from build123d import *

# Parameters (mm, degrees)
SKETCH1_R           = 28.575
SKETCH1_R_2         = 12.7
SKETCH1_R_3         = 3.175
BOSS_EXTRUDE1_DEPTH = 6.35


with BuildPart() as part:
    # Sketch1 → Boss-Extrude1 (new body)
    with BuildSketch(Plane.ZY.offset(-33.3375)):
        with Locations((-3.206573009, 186.931527045)):
            Circle(SKETCH1_R)
        with Locations((-3.206573009, 186.931527045)):
            Circle(SKETCH1_R_2, mode=Mode.SUBTRACT)
        with Locations((19.018426991, 186.931527045)):
            Circle(SKETCH1_R_3, mode=Mode.SUBTRACT)
        with Locations((-3.206573009, 164.706527045)):
            Circle(SKETCH1_R_3, mode=Mode.SUBTRACT)
        with Locations((-25.431573009, 186.931527045)):
            Circle(SKETCH1_R_3, mode=Mode.SUBTRACT)
        with Locations((-3.206573009, 209.156527045)):
            Circle(SKETCH1_R_3, mode=Mode.SUBTRACT)
    extrude(amount=BOSS_EXTRUDE1_DEPTH)


solid = part.part
For this review, take the finished solid that the model builds, in its own axes (mm). Round coordinates to 2 decimals unless told otherwise and drop trailing zeros. Write each loop counter-clockwise with the first axis right and the second up, starting at its lowest first coordinate (ties: lowest second). Pieces come first, ordered by that corner, then holes. Notation, with made-up numbers: M 41.25,12 L 76.25,12 A27 cw 76.25,50 Z; hole C -36.5,21.25 d3. An arc over 180 degrees is marked long. Write item = value, one per line. Start each with the question number.
(1) We need section D-D (x = 29.5). Give the boundary of the cut face in (y, z) (3 decimals), then the cut area to 3 significant figures.
(2) The part is to be moulded in two halves that separate along Z. For faces 1 (the face through (33.338, 175, 3)), 2 (the face through (30.207, 211.026, 12.155)), 3 (the face through (30.207, 187.885, 22.047)), say which applies: +Z half, -Z half, draft (parallel to the pull), parting line (faces both ways), or undercut.
(3) For line 1 along Y through (x, z) = (29.5, -2.5); line 2 along Z through (x, y) = (30.75, 188); line 3 along Z through (x, y) = (31.25, 190.5), list the stretches that pass through material, from the lowest coordinate up.
(4) We need section C-C (z = 19.5). Give the boundary of the cut face in (x, y).
(5) Clearance check with flat-ended pins moving along their axes: pin 1 Ø1.5 at (x, y) = (30.5, 192.5) entering from +Z; pin 2 Ø1.5 at (x, z) = (29.5, 9.5) entering from -Y. State where each tip first meets the part, or that it passes through.
(6) We need section A-A (z = -3.5). Give the boundary of the cut face in (x, y).
(7) We need section B-B (y = 167). Give the boundary of the cut face in (x, z).
Results found:
q1.outline = C 186.932,-3.207 d57.15; hole C 164.707,-3.207 d6.35; hole C 186.932,-3.207 d25.4; hole C 186.932,-25.432 d6.35; hole C 186.932,19.018 d6.35; hole C 209.157,-3.207 d6.35
q1.area = 1,930 mm²
q2.face_1 = draft
q2.face_2 = parting line
q2.face_3 = undercut
q3.line_1 = 158.37 to 161.61, 167.8 to 174.25, 199.61 to 206.06, 212.25 to 215.5
q3.line_2 = -31.76 to -28.42, -22.44 to -15.86, 9.45 to 16.03, 22.01 to 25.35
q3.line_3 = -31.56 to -15.39, 8.98 to 25.14
q4.outline = M 26.99,169.58 L 33.34,169.58 L 33.34,183.79 L 26.99,183.79 Z; M 26.99,190.07 L 33.34,190.07 L 33.34,204.28 L 26.99,204.28 Z
q5.pin_1 = 24.96
q5.pin_2 = 160.98
q6.outline = M 26.99,158.36 L 33.34,158.36 L 33.34,161.55 L 26.99,161.55 Z; M 26.99,167.87 L 33.34,167.87 L 33.34,174.23 L 26.99,174.23 Z; M 26.99,199.63 L 33.34,199.63 L 33.34,206 L 26.99,206 Z; M 26.99,212.32 L 33.34,212.32 L 33.34,215.51 L 26.99,215.51 Z
q7.outline = M 26.99,-23.68 L 33.34,-23.68 L 33.34,-5.4 L 26.99,-5.4 Z; M 26.99,-1.01 L 33.34,-1.01 L 33.34,17.27 L 26.99,17.27 Z
